For this review, take the finished solid that the model builds, in its own axes (mm). Round coordinates to 2 decimals unless told otherwise and drop trailing zeros. Loops run counter-clockwise (first coordinate to the right, second up) from the corner with the lowest first, then second, coordinate; pieces in that order, holes last.
1) Take a section at C-C (y = 1576.5). State the section outline as (x, z) points, then the cut area to 3 significant figures.
2) Take a section at B-B (z = 2.5). State the section outline as (x, y) points.
3) Insertion check: pin 1 (2 mm diameter, centred on x = 670, z = 4.5, fed in from +Y); pin 2 (6 mm diameter, centred on x = 679.5, z = 3.5, fed in from -Y); pin 3 (4 mm diameter, centred on x = 693, z = 7, fed in from +Y). Each pin has a flat end and moves straight along its axis. Give the tip position at first contact, or say it passes through.
4) Take a section at A-A (x = 789.5). State the section outline as (y, z) points.
5) Wall thickness on L1, parallel to X at y = 1663, z = 8.75; L2, parallel to X at y = 1598, z = 4.5; L3, parallel to Y at x = 688, z = 1: over which ranges is each line inside the solid? List them lowest first.
Autodesk Inventor part; units mm, degrees
ref_plane "YZ Plane" through (0, 0, 0) normal (1, 0, 0) x (0, 1, 0)
ref_plane "XZ Plane" through (0, 0, 0) normal (0, 1, 0) x (-1, 0, 0)
ref_plane "XY Plane" through (0, 0, 0) normal (0, 0, 1) x (1, 0, 0)
sketch "Sketch1" plane through (0, 0, 0) normal (0, 0, 1) x (1, 0, 0)
  arc A0 (763.7742, 1811.2181) -> (637.7742, 1685.2181) centre (763.7742, 1685.2181) ccw
  arc A1 (763.7742, 1791.2181) -> (657.7742, 1685.2181) centre (763.7742, 1685.2181) ccw
  line L0 (637.7742, 1546.2181) -> (657.7742, 1546.2181)
  circle A2 centre (763.7742, 1801.2181) radius 3.5
  circle A3 centre (647.7742, 1596.2181) radius 3.5
  circle A4 centre (647.7742, 1685.2181) radius 3.5
  line L1 (802.7742, 1811.2181) -> (802.7742, 1791.2181)
  circle A5 centre (681.7499, 1767.2425) radius 3.5
  line L2 (637.7742, 1685.2181) -> (637.7742, 1546.2181)
  line L3 (657.7742, 1546.2181) -> (657.7742, 1685.2181)
  line L4 (763.7742, 1791.2181) -> (802.7742, 1791.2181)
  line L5 (802.7742, 1811.2181) -> (763.7742, 1811.2181)
  point P0 (0, 0)
extrude "Extrusion1" add sketch "Sketch1" along normal blind 10
properties part number "side_walls"
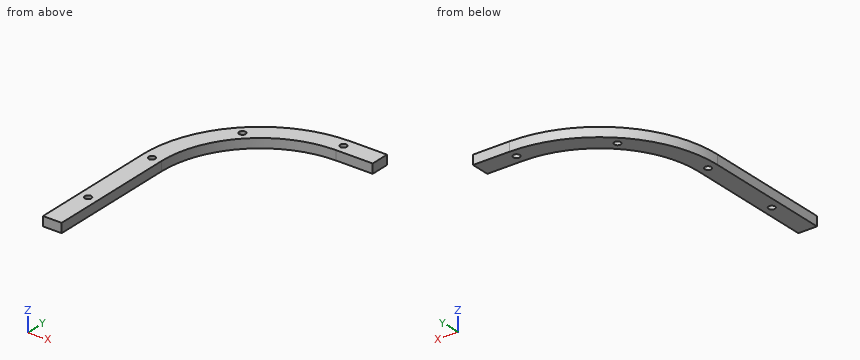
Response:
1. outline: (637.77, 0) - (657.77, 0) - (657.77, 10) - (637.77, 10) - close
1. area: 200 mm2
2. outline: (637.77, 1546.22) - (657.77, 1546.22) - (657.77, 1685.22) arc R106 cw to (763.77, 1791.22) - (802.77, 1791.22) - (802.77, 1811.22) - (763.77, 1811.22) arc R126 ccw to (637.77, 1685.22) - close; hole circle Ø7 at (647.77, 1596.22); hole circle Ø7 at (647.77, 1685.22); hole circle Ø7 at (681.75, 1767.24); hole circle Ø7 at (763.77, 1801.22)
3. pin 1: stops at y = 1770.48
3. pin 2: stops at y = 1745.38
3. pin 3: stops at y = 1790.79
4. outline: (1791.22, 0) - (1811.22, 0) - (1811.22, 10) - (1791.22, 10) - close
5. L1: x = 637.77 to 657.77
5. L2: x = 637.77 to 644.76, 650.79 to 657.77
5. L3: y = 1759.34 to 1785.89
